```python
from build123d import *

# Parameters (mm, degrees)
SKETCH1_R           = 11
BOSS_EXTRUDE1_DEPTH = 3.6
SKETCH2_R           = 5
BOSS_EXTRUDE2_DEPTH = 10
BOSS_EXTRUDE3_START = 1.5
SKETCH3_R           = 5
BOSS_EXTRUDE3_DEPTH = 1.5
SKETCH4_R           = 4
CUT_EXTRUDE1_DEPTH  = 22.67971402
SKETCH5_R           = 1.5
CUT_EXTRUDE2_DEPTH  = 19.493242009
CIRPATTERN1_COUNT   = 4


with BuildPart() as part:
    # Sketch1 → Boss-Extrude1 (new body)
    with BuildSketch(Plane(origin=(0, 0, 0), x_dir=(1, 0, 0), z_dir=(0, 1, 0))):
        with Locations(Location((0, 0, 0), (0, 0, 270))):
            Circle(SKETCH1_R)
    extrude(amount=BOSS_EXTRUDE1_DEPTH)

    # Sketch2 → Boss-Extrude2 (add)
    with BuildSketch(Plane(origin=(0, 3.6, 0), x_dir=(1, 0, 0), z_dir=(0, 1, 0))):
        with Locations(Location((0, 0, 0), (0, 0, 270))):
            Circle(SKETCH2_R)
    extrude(amount=BOSS_EXTRUDE2_DEPTH)

    # Sketch3 → Boss-Extrude3 (add)
    with BuildSketch(Plane.XZ.offset(BOSS_EXTRUDE3_START)):
        with Locations(Location((0, 0, 0), (0, 0, 90))):
            Circle(SKETCH3_R)
    extrude(amount=-BOSS_EXTRUDE3_DEPTH)

    # Sketch4 → Cut-Extrude1 (cut, through all)
    with BuildSketch(Plane(origin=(0, 13.6, 0), x_dir=(1, 0, 0), z_dir=(0, 1, 0))):
        with Locations(Location((0, 0, 0), (0, 0, 270))):
            Circle(SKETCH4_R)
    extrude(amount=-CUT_EXTRUDE1_DEPTH, mode=Mode.SUBTRACT)

    # Sketch5 → Cut-Extrude2 (cut, symmetric)
    with BuildSketch(Plane(origin=(0, 3.6, 0), x_dir=(1, 0, 0), z_dir=(0, 1, 0))):
        with Locations(Location((0, 8, 0), (0, 0, 270))):
            Circle(SKETCH5_R)
    cut_extrude2 = extrude(amount=CUT_EXTRUDE2_DEPTH, both=True, mode=Mode.SUBTRACT)

    # CirPattern1: Cut-Extrude2 ×4 about axis
    cirpattern1_axis = Axis((0, 0, 0), (0, 1, 0))
    for i in range(1, CIRPATTERN1_COUNT):
        add(cut_extrude2.rotate(cirpattern1_axis, i * 360 / CIRPATTERN1_COUNT), mode=Mode.SUBTRACT)


solid = part.part
```
Build history of the part. All positions in model axes, mm. A direction names the side the tool comes from. Give positions to 0.01 mm unless a question says otherwise; leave off trailing zeros. Loops run counter-clockwise (first coordinate to the right, second up) from the corner with the lowest first, then second, coordinate; pieces in that order, holes last.
Item 1: Drill centre lines: line 1 (X direction, y = 6.5, z = 0); line 2 (Z direction, x = 8, y = 0.8); line 3 (X direction, y = 1.25, z = -8.75). Where is each one in solid material? Low to high.
Answers follow:
line 1: x = -5 to -4, 4 to 5
line 2: z = -7.55 to -1.5, 1.5 to 7.55
line 3: x = -6.67 to -1.3, 1.3 to 6.67
Item 2: Slice it at A-A, the plane z = 0. List the corners of the cut face in (x, y).
Answers follow:
outline: (-11, 0) - (-9.5, 0) - (-9.5, 3.6) - (-11, 3.6) - close; (-6.5, 0) - (-5, 0) - (-5, -1.5) - (-4, -1.5) - (-4, 13.6) - (-5, 13.6) - (-5, 3.6) - (-6.5, 3.6) - close; (4, -1.5) - (5, -1.5) - (5, 0) - (6.5, 0) - (6.5, 3.6) - (5, 3.6) - (5, 13.6) - (4, 13.6) - close; (9.5, 0) - (11, 0) - (11, 3.6) - (9.5, 3.6) - close
Item 3: Which spindle directions (+Z, -Z, +X, -X, +Y, -Y) get a long thin tool onto all of the face, cutting with end or side? Do faces 1 (the face through (-4.88, 8.53, -1.08)), 2 (the face through (4.88, -0.76, -1.08)), 3 (the face through (0.07, 1.83, -9.5)). Say none if no direction does.
Answers follow:
face 1: +Y
face 2: -Y
face 3: +Y, -Y
Item 4: Flat gauge pins, fed straight in: pin 1 (2.5 mm diameter, centred on x = 8, z = 0, fed in from -Y); pin 2 (4 mm diameter, centred on x = 0, z = 8, fed in from -Y); pin 3 (8 mm diameter, centred on x = 1.5, y = 10, fed in from +Z); pin 4 (5 mm diameter, centred on y = 7, z = -5.5, fed in from +X). Where does each tip first touch, or does it go through?
Answers follow:
pin 1: passes through
pin 2: stops at y = 0
pin 3: stops at z = 5
pin 4: stops at x = 4
Item 5: Pull direction Z, two halves, no side cores. Call faces 4 (the face through (-5, 3.6, 2)), 5 (the face through (-10.74, 1.77, -2.38)), 6 (the face through (-3.905, 6.156, -0.867)): released by +Z, released by -Z, zero draft, split by the parting line, or undercut.
Answers follow:
face 4: zero draft
face 5: split by the parting line
face 6: undercut
Item 6: Slice it at B-B, the plane x = -7. List the corners of the cut face in (y, z), and give its area (3 significant figures).
Answers follow:
outline: (0, -8.49) - (3.6, -8.49) - (3.6, -1.12) - (0, -1.12) - close; (0, 1.12) - (3.6, 1.12) - (3.6, 8.49) - (0, 8.49) - close
area: 53.0 mm2
Item 7: Slice it at D-D, the plane z = 8. List the corners of the cut face in (x, y), and give its area (3 significant figures).
Answers follow:
outline: (-7.55, 0) - (-1.5, 0) - (-1.5, 3.6) - (-7.55, 3.6) - close; (1.5, 0) - (7.55, 0) - (7.55, 3.6) - (1.5, 3.6) - close
area: 43.6 mm2
Item 8: Slice it at C-C, the plane y = 1.75. List the corners of the cut face in (x, z), and give its area (3 significant figures).
Answers follow:
outline: circle Ø22 at (0, 0); hole circle Ø3 at (-8, 0); hole circle Ø8 at (0, 0); hole circle Ø3 at (0, -8); hole circle Ø3 at (0, 8); hole circle Ø3 at (8, 0)
area: 302 mm2
